from build123d import *

# Parameters (mm, degrees)
EXTRUDE_1_DEPTH     = 4
SKETCH_3_R          = 10.969655115
EXTRUDE_2_DEPTH     = 2
SKETCH_4_R          = 7.5
CUT_EXTRUDE_1_DEPTH = 17.633299933


with BuildPart() as part:
    # Sketch 1 → Extrude 1 (new body)
    with BuildSketch(Plane(origin=(0, 0, 0), x_dir=(1, 0, 0), z_dir=(0, 1, 0))):
        Polygon((-5.484827557, 9.5), (5.484827557, 9.5), (10.969655115, 0), (5.484827557, -9.5), (-5.484827557, -9.5), (-10.969655115, 0), align=None)
    extrude(amount=EXTRUDE_1_DEPTH)

    # Sketch 3 → Extrude 2 (add)
    with BuildSketch(Plane.XZ):
        with Locations(Location((0, 0, 0), (0, 0, 120))):
            Circle(SKETCH_3_R)
    extrude(amount=EXTRUDE_2_DEPTH)

    # Sketch 4 → Cut-Extrude 1 (cut, through all)
    with BuildSketch(Plane.XZ.offset(2)):
        with Locations(Location((0, 0, 0), (0, 0, 270))):
            Circle(SKETCH_4_R)
    extrude(amount=-CUT_EXTRUDE_1_DEPTH, mode=Mode.SUBTRACT)


solid = part.part
Design review of the part built by this model. Coordinates are the model's own, in mm. A direction names the side the tool comes from. Round coordinates to 2 decimals unless told otherwise and drop trailing zeros. Write each loop counter-clockwise with the first axis right and the second up, starting at its lowest first coordinate (ties: lowest second). Pieces come first, ordered by that corner, then holes.
Item 1: Consider section B-B on x = 0. Give the boundary of the cut face in (y, z).
Item 2: Wall thickness on L1, parallel to Z at x = 3, y = 3.5; L2, parallel to Z at x = 5, y = -0.6; L3, parallel to X at y = 2.2, z = 6.25: over which ranges is each line inside the solid? List them lowest first.
Item 3: For pin 1 Ø2 at (x, y) = (6.5, -1) entering from +Z; pin 2 Ø1.2 at (x, z) = (0, -10.5) entering from +Y; pin 3 Ø1.2 at (x, z) = (-2.5, 10) entering from +Y; pin 4 Ø3 at (x, y) = (-1.5, 2) entering from -Z, all flat-tipped, find the tip position at first contact; note any pin that passes through.
Item 4: Draft analysis for pull direction X (two halves, no side actions). For faces 4 (the flat face through (-8.266, 1.972, -4.684)), 5 (the cylindrical face through (10.463, -0.986, 3.295)), 6 (the flat face through (9, 0, 5)), 7 (the cylindrical face through (0.33, 0.958, 7.493)), state which applies: released by +X, released by -X, zero draft, split by the parting line, or undercut.
Item 5: Consider section A-A on y = 1.2. Give the boundary of the cut face in (x, z).
Item 6: For faces 1 (the flat face through (0, 0, -10)), 2 (the flat face through (-8.2, 2, 4.8)), 3 (the flat face through (9, 0, -5)), list the 3-axis set-ups (+Z, -Z, +X, -X, +Y, -Y) from which the entire face can be reached by the end or side of a thin tool; tool diameter is ignored.
Item 7: Consider section C-C on z = 5.25. Give the boundary of the cut face in (x, y), and give its area (3 significant figures).
Check values:
1. outline: (-2, -10.97) - (0, -10.97) - (0, -9.5) - (4, -9.5) - (4, -7.5) - (-2, -7.5) - close; (-2, 7.5) - (4, 7.5) - (4, 9.5) - (0, 9.5) - (0, 10.97) - (-2, 10.97) - close
2. L1: z = -9.5 to -6.87, 6.87 to 9.5
2. L2: z = -9.76 to -5.59, 5.59 to 9.76
2. L3: x = -7.36 to -4.15, 4.15 to 7.36
3. pin 1: stops at z = 9.49
3. pin 2: stops at y = 0
3. pin 3: stops at y = 4
3. pin 4: stops at z = -9.5
4. face 4: released by -X
4. face 5: split by the parting line
4. face 6: zero draft
4. face 7: undercut
5. outline: (-10.97, 0) - (-5.48, -9.5) - (5.48, -9.5) - (10.97, 0) - (5.48, 9.5) - (-5.48, 9.5) - close; hole circle Ø15 at (0, 0)
6. face 1: -Z, +X, -X, +Y
6. face 2: +Z, -X, +Y
6. face 3: -Z, +X, +Y
7. outline: (-9.63, -2) - (-5.36, -2) - (-5.36, 4) - (-7.94, 4) - (-7.94, 0) - (-9.63, 0) - close; (5.36, -2) - (9.63, -2) - (9.63, 0) - (7.94, 0) - (7.94, 4) - (5.36, 4) - close
7. area: 37.8 mm2
